Design review of the part built by this model. Coordinates are the model's own, in mm. Face numbers are marked on the shaded views. A direction names the side the tool comes from. Coordinates: 2 decimals unless noted, no trailing zeros. Write each loop counter-clockwise with the first axis right and the second up, starting at its lowest first coordinate (ties: lowest second). Pieces come first, ordered by that corner, then holes. Notation, with made-up numbers: M 70,25 L 75,25 A29 cw 75,58 Z; hole C 47.5,32.25 d10. An arc over 180 degrees is marked long. Write each question's results on one line, items separated by ' | '. Start each with the question number.
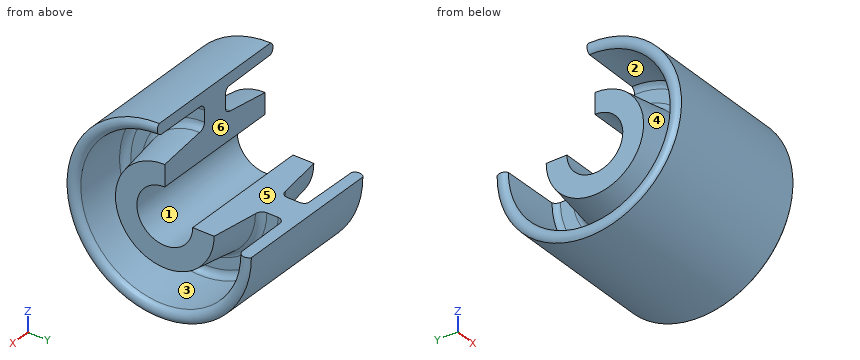
```python
from build123d import *

# Parameters (mm, degrees)
REVOLVE2_ANGLE = 270


with BuildPart() as part:
    # Sketch1 → Revolve2 (revolve)
    with BuildSketch(Plane.XY):
        with BuildLine():
            Line((-50.632149816, 30.528207977), (29.367850184, 30.528207977))
            ThreePointArc((29.367850184, 30.528207977), (30.674979125, 26.908813233), (27.867850184, 24.276583855))
            Line((27.867850184, 24.276583855), (0.367850184, 24.028207977))
            ThreePointArc((0.367850184, 24.028207977), (-2.10702355, 23.003081711), (-3.132149816, 20.528207977))
            Line((-3.132149816, 20.528207977), (-3.132149816, 14.528207977))
            ThreePointArc((-3.132149816, 14.528207977), (-2.10702355, 12.053334243), (0.367850184, 11.028207977))
            Line((0.367850184, 11.028207977), (25.367850184, 7.528207977))
            Line((25.367850184, 7.528207977), (25.367850184, -3.971792023))
            Line((25.367850184, -3.971792023), (-46.632149816, -3.971792023))
            Line((-46.632149816, -3.971792023), (-46.632149816, 7.190485637))
            Line((-46.632149816, 7.190485637), (-21.632149816, 10.690485637))
            ThreePointArc((-21.632149816, 10.690485637), (-19.157276082, 11.715611903), (-18.132149816, 14.190485637))
            Line((-18.132149816, 14.190485637), (-18.132149816, 20.865930317))
            ThreePointArc((-18.132149816, 20.865930317), (-18.642058581, 22.685093423), (-20.023209476, 23.974195264))
            Line((-20.023209476, 23.974195264), (-50.632149816, 24.505975141))
            ThreePointArc((-50.632149816, 24.505975141), (-52.348003545, 27.517091559), (-50.632149816, 30.528207977))
        make_face()
    revolve(axis=Axis((35.391313148, -18.971792023, 0), (-1, 0, 0)), revolution_arc=REVOLVE2_ANGLE)


solid = part.part
```
Item 1: Draft analysis for pull direction Y (two halves, no side actions). For the marked faces 4, 5 and 6, state which applies: released by +Y, released by -Y, zero draft, split by the parting line, or undercut.
Item 2: Insertion check: pin 1 Ø5 at (x, z) = (-32, 37) entering from +Y; pin 2 Ø5 at (x, z) = (9.5, -29.5) entering from -Y; pin 3 Ø1.5 at (x, z) = (-21, 12.5) entering from +Y. Each pin has a flat end and moves straight along its axis. Give the tip position at first contact, or say it passes through.
Item 3: We need section C-C on x = -34. State the section outline as (y, z) points.
Item 4: Wall thickness on L1, parallel to Z at x = -29.5, y = -38.5; L2, parallel to Y at x = -33, z = 13.5; L3, parallel to X at y = -15, z = -33: over which ranges is each line inside the solid? List them lowest first.
Item 5: For the marked faces 1, 2 and 3, list the 3-axis set-ups (+Z, -Z, +X, -X, +Y, -Y) from which the entire face can be reached by the end or side of a thin tool; tool diameter is ignored.
Item 6: We need section A-A on x = 17. State the section outline as (y, z) points.
Item 7: We need section B-B on x = -8.5. State the section outline as (y, z) points.
Answer:
1) face 4: undercut | face 5: zero draft | face 6: released by +Y
2) pin 1: stops at y = -36.35 | pin 2: stops at y = -60.46 | pin 3: stops at y = -26
3) outline: M -18.97,15 L -18.97,27.93 A27.93 ccw long 8.96,0 L -3.97,0 A15 cw long Z; M -18.97,43.19 L -18.97,49.5 A49.5 ccw long 30.53,0 L 24.22,0 A43.19 cw long Z
4) L1: z = -45.49 to -38.43, -20.84 to 20.84, 38.43 to 45.49 | L2: y = -66.6 to -59.98, -43.58 to -25.51 | L3: x = -18.13 to -3.12
5) face 1: +X, -X | face 2: -X | face 3: +X
6) outline: M -18.97,15 L -18.97,27.67 A27.67 ccw long 8.7,0 L -3.97,0 A15 cw long Z; M -18.97,43.15 L -18.97,49.5 A49.5 ccw long 30.53,0 L 24.18,0 A43.15 cw long Z
7) outline: M -18.97,15 L -18.97,49.5 A49.5 ccw long 30.53,0 L -3.97,0 A15 cw long Z
